Can you work these out from the drawing? Everything is in mm from the part's minimum corner. Give positions to 0.01 mm unless a question says otherwise; leave off trailing zeros. Loops run counter-clockwise (first coordinate to the right, second up) from the corner with the lowest first, then second, coordinate; pieces in that order, holes last. Notation, with made-up numbers: (69, 13) - (80, 13) arc R25 ccw to (80, 45) - close; hole circle Ø2 at (51, 11). An arc over 180 degrees is marked (long way). Answer in a Markdown table with one row per item. Add a question column.
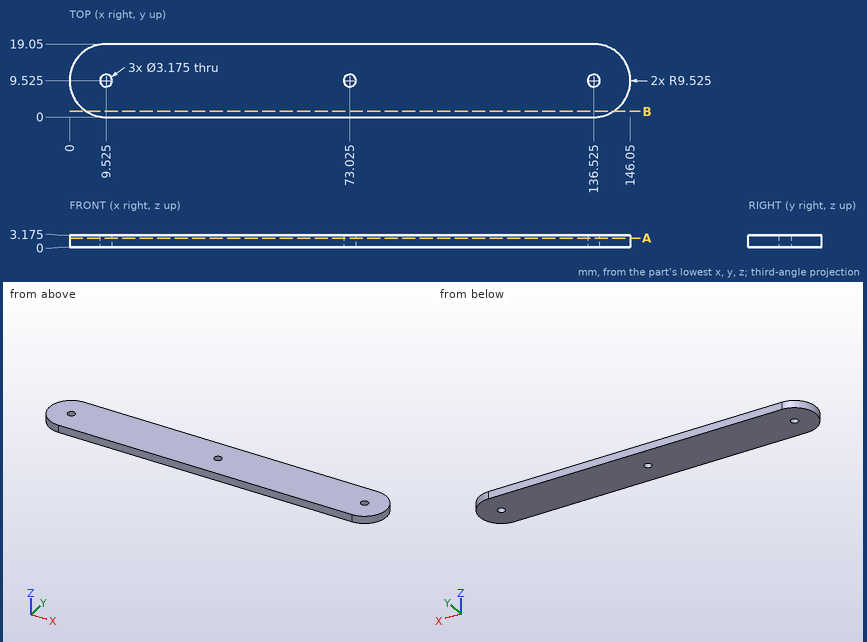
(1) For pin 1 Ø1.9 at (x, y) = (73.025, 9.525) entering from -Z; pin 2 Ø4 at (x, y) = (9.525, 9.525) entering from -Z, each with a flat end and sliding along its axis, tell me the tip position at first contact or that it passes through.
(2) I want a section at B-B on y = 1.5. Please give me the cut outline in (x, z) (3 decimals).
(3) I want a section at A-A on z = 2.4. State how many separate pieces and enclosed holes the cut face has, then the cut area to 3 significant figures.
(4) Please list where these lines run through material, in increasing order: line 1 (X direction, y = 8.25, z = 1.3); line 2 (X direction, y = 10.5, z = 1.6); line 3 (Y direction, x = 136, z = 0.45).
Reported:
| question | item | result |
|---|---|---|
| 1 | pin 1 | through |
| 1 | pin 2 | z = 0 |
| 2 | outline | (4.394, 0) - (141.656, 0) - (141.656, 3.175) - (4.394, 3.175) - close |
| 3 | separate pieces | 1 |
| 3 | enclosed holes | 3 |
| 3 | area | 2,680 mm² |
| 4 | line 1 | 0.09 to 8.58, 10.47 to 72.08, 73.97 to 135.58, 137.47 to 145.96 |
| 4 | line 2 | 0.05 to 8.27, 10.78 to 71.77, 74.28 to 135.27, 137.78 to 146 |
| 4 | line 3 | 0 to 8.03, 11.02 to 19.05 |
